from build123d import *

# Parameters (mm, degrees)
ESQUISSE1_R        = 3
BOSS_EXTRU_1_DEPTH = 16
CHANFREIN1_SIZE    = 0.5


with BuildPart() as part:
    # Esquisse1 → Boss.-Extru.1 (new body)
    with BuildSketch(Plane(origin=(0, 0, 0), x_dir=(1, 0, 0), z_dir=(0, 1, 0))):
        Circle(ESQUISSE1_R)
    extrude(amount=BOSS_EXTRU_1_DEPTH)

    # Esquisse4 → Révolution1 (revolve)
    with BuildSketch(Plane(origin=(0, 0, 0), x_dir=(0, 0, -1), z_dir=(1, 0, 0))):
        with BuildLine():
            Line((0, 0), (28, 0))
            Line((28, 0), (28, -1))
            ThreePointArc((28, -1), (26, -3), (28, -5))
            Line((28, -5), (28, -6))
            Line((28, -6), (0, -6))
            Line((0, -6), (0, 0))
        make_face()
    revolve(axis=Axis((0, -6, 0), (0, 1, 0)))

    # Chanfrein1
    chanfrein1_edges = [part.edges().sort_by_distance(p)[0] for p in [
        (-3, 16, 0),
    ]]
    chamfer(chanfrein1_edges, length=CHANFREIN1_SIZE)


solid = part.part
Verification items for the finished model (mm, model axes). A direction names the side the tool comes from. Coordinates: 2 decimals unless noted, no trailing zeros. Write each loop counter-clockwise with the first axis right and the second up, starting at its lowest first coordinate (ties: lowest second). Pieces come first, ordered by that corner, then holes. Notation, with made-up numbers: (85, -35) -> (92, -35) arc R8 ccw to (92, -23) -> close; hole circle Ø6 at (70, -39). An arc over 180 degrees is marked (long way). One line per item, written item: value. Start each with the question number.
Q1. Cross-section at C-C on y = 7.75. Enter the section's corners in (x, z).
Q2. Cross-section at A-A on x = 0. Enter the section's corners in (y, z).
Q3. Cross-section at B-B on z = 0. Enter the section's corners in (x, y).
Q4. Thickness scan on L1, parallel to Y at x = 17.5, z = -15.5; L2, parallel to Y at x = 24.5, z = -12; L3, parallel to Z at x = -19, y = -3. Record the ranges inside material, lowest first. Write a range as from..to.
Q5. Access from +Z, -Z, +X, -X, +Y, -Y to the whole of each face (thin tool, end or side, straight path). Record for faces 1 (the cylindrical face through (-3, 8, 0)), 2 (the cylindrical face through (10.724, -5.507, -25.865)).
Q6. Go/stop test with flat-tipped pins: P1, Ø12, axis at y = 3, z = -10, coming from the +X side; P2, Ø1.5, axis at x = 16.5, y = 0, coming from the -Z side; P3, Ø2, axis at x = -6, z = -1, coming from the +Y side; P4, Ø3, axis at x = 7, y = 2, coming from the +Z side. Record where each tip stops, or that it passes through.
Checked values:
1. outline: circle Ø6 at (0, 0)
2. outline: (-6, -28) -> (-5, -28) arc R2 cw to (-1, -28) -> (0, -28) -> (0, -3) -> (15.5, -3) -> (16, -2.5) -> (16, 2.5) -> (15.5, 3) -> (0, 3) -> (0, 28) -> (-1, 28) arc R2 cw to (-5, 28) -> (-6, 28) -> close
3. outline: (-28, -6) -> (28, -6) -> (28, -5) arc R2 cw to (28, -1) -> (28, 0) -> (3, 0) -> (3, 15.5) -> (2.5, 16) -> (-2.5, 16) -> (-3, 15.5) -> (-3, 0) -> (-28, 0) -> (-28, -1) arc R2 cw to (-28, -5) -> close
4. L1: y = -6..0
4. L2: y = -6..-4.87, -1.13..0
4. L3: z = -17.75..17.75
5. face 1: +Y
5. face 2: +Y, -Y
6. P1: stops at x = 27.58
6. P2: stops at z = -23.15
6. P3: stops at y = 0
6. P4: passes through
